Autodesk Fusion 360 part; units mm, degrees
sketch "Sketch1" plane through (0, 0, 0) normal (0, 0, 1) x (1, 0, 0)
  line L0 (0, 0) -> (28, 0)
  line L1 (28, 0) -> (28, 160)
  line L2 (28, 160) -> (0, 160)
  line L3 (0, 160) -> (0, 0) construction
  line L4 (20, 0) -> (20, 160) construction
  line L5 (22.5, 155) -> (25.5, 155)
  line L6 (25.5, 155) -> (25.5, 145)
  line L7 (25.5, 145) -> (22.5, 145)
  line L8 (22.5, 145) -> (22.5, 155)
  line L9 (25.5, 155) -> (25.5, 160) construction
  line L10 (25.5, 155) -> (28, 155) construction
  line L11 (22.5, 135) -> (25.5, 135)
  line L12 (25.5, 135) -> (25.5, 125)
  line L13 (25.5, 125) -> (22.5, 125)
  line L14 (22.5, 125) -> (22.5, 135)
  line L15 (24, 145) -> (24, 135) construction
  line L16 (22.5, 105) -> (22.5, 115)
  line L17 (25.5, 105) -> (22.5, 105)
  line L18 (25.5, 115) -> (25.5, 105)
  line L19 (22.5, 115) -> (25.5, 115)
  line L20 (24, 115) -> (24, 125) construction
  line L21 (25.5, 95) -> (25.5, 85)
  line L22 (25.5, 85) -> (22.5, 85)
  line L23 (22.5, 85) -> (22.5, 95)
  line L24 (22.5, 95) -> (25.5, 95)
  line L25 (24, 95) -> (24, 105) construction
  line L26 (25.5, 95) -> (28, 95) construction
  line L27 (22.5, 75) -> (25.5, 75)
  line L28 (25.5, 75) -> (25.5, 65)
  line L29 (25.5, 65) -> (22.5, 65)
  line L30 (22.5, 65) -> (22.5, 75)
  line L31 (22.5, 55) -> (25.5, 55)
  line L32 (25.5, 55) -> (25.5, 45)
  line L33 (25.5, 45) -> (22.5, 45)
  line L34 (22.5, 45) -> (22.5, 55)
  line L35 (24, 85) -> (24, 75) construction
  line L36 (25.5, 75) -> (28, 75) construction
  line L37 (25.5, 55) -> (28, 55) construction
  line L38 (24, 55) -> (24, 65) construction
  line L39 (25.5, 135) -> (28, 135) construction
  line L40 (25.5, 115) -> (28, 115) construction
  line L41 (22.5, 35) -> (25.5, 35)
  line L42 (25.5, 35) -> (25.5, 25)
  line L43 (25.5, 25) -> (22.5, 25)
  line L44 (22.5, 25) -> (22.5, 35)
  line L45 (25.5, 35) -> (28, 35) construction
  line L46 (24, 45) -> (24, 35) construction
  line L47 (22.5, 15) -> (25.5, 15)
  line L48 (25.5, 15) -> (25.5, 5)
  line L49 (25.5, 5) -> (22.5, 5)
  line L50 (22.5, 5) -> (22.5, 15)
  line L51 (24, 15) -> (24, 25) construction
  line L52 (25.5, 15) -> (28, 15) construction
  line L53 (-25.5, 75) -> (-28, 75) construction
  line L54 (-25.5, 75) -> (-25.5, 65)
  line L55 (-20, 0) -> (-20, 160) construction
  line L56 (-24, 85) -> (-24, 75) construction
  line L57 (-25.5, 115) -> (-28, 115) construction
  line L58 (-22.5, 45) -> (-22.5, 55)
  line L59 (-25.5, 145) -> (-22.5, 145)
  line L60 (-25.5, 135) -> (-28, 135) construction
  line L61 (-22.5, 115) -> (-25.5, 115)
  line L62 (-25.5, 105) -> (-22.5, 105)
  line L63 (-22.5, 65) -> (-22.5, 75)
  line L64 (0, 160) -> (0, 0) construction
  line L65 (-24, 45) -> (-24, 35) construction
  line L66 (-25.5, 135) -> (-25.5, 125)
  line L67 (-28, 160) -> (0, 160)
  line L68 (-25.5, 155) -> (-28, 155) construction
  line L69 (-25.5, 125) -> (-22.5, 125)
  line L70 (-25.5, 55) -> (-28, 55) construction
  line L71 (-24, 15) -> (-24, 25) construction
  line L72 (-22.5, 135) -> (-25.5, 135)
  line L73 (-25.5, 15) -> (-28, 15) construction
  line L74 (-22.5, 75) -> (-25.5, 75)
  line L75 (-25.5, 115) -> (-25.5, 105)
  line L76 (-25.5, 155) -> (-25.5, 145)
  line L77 (-22.5, 105) -> (-22.5, 115)
  line L78 (-24, 115) -> (-24, 125) construction
  line L79 (-25.5, 95) -> (-25.5, 85)
  line L80 (-25.5, 55) -> (-25.5, 45)
  line L81 (-28, 0) -> (-28, 160)
  line L82 (-22.5, 155) -> (-25.5, 155)
  line L83 (-22.5, 85) -> (-22.5, 95)
  line L84 (-24, 95) -> (-24, 105) construction
  line L85 (-25.5, 15) -> (-25.5, 5)
  line L86 (-25.5, 5) -> (-22.5, 5)
  line L87 (-25.5, 155) -> (-25.5, 160) construction
  line L88 (-25.5, 35) -> (-28, 35) construction
  line L89 (-22.5, 25) -> (-22.5, 35)
  line L90 (-22.5, 35) -> (-25.5, 35)
  line L91 (-25.5, 95) -> (-28, 95) construction
  line L92 (-25.5, 25) -> (-22.5, 25)
  line L93 (-22.5, 95) -> (-25.5, 95)
  line L94 (-25.5, 45) -> (-22.5, 45)
  line L95 (-22.5, 125) -> (-22.5, 135)
  line L96 (-22.5, 145) -> (-22.5, 155)
  line L97 (-24, 145) -> (-24, 135) construction
  line L98 (-22.5, 55) -> (-25.5, 55)
  line L99 (-25.5, 65) -> (-22.5, 65)
  line L100 (-25.5, 85) -> (-22.5, 85)
  line L101 (-24, 55) -> (-24, 65) construction
  line L102 (-25.5, 35) -> (-25.5, 25)
  line L103 (0, 0) -> (-28, 0)
  line L104 (-22.5, 15) -> (-25.5, 15)
  line L105 (-22.5, 5) -> (-22.5, 15)
  point P0 (24, 115)
  point P1 (24, 95)
  point P2 (24, 95)
  point P3 (-24, 115)
  point P4 (-24, 95)
  point P5 (-24, 95)
  dimension "d3" = 160
  dimension "d4" = 28
  dimension "d5" = 5
  dimension "d6" = 2.5
  dimension "d7" = 10
  dimension "d8" = 3
  dimension "d9" = 10
extrude "Extrude1" add sketch "Sketch1" along normal blind 3
sketch "Sketch2" plane through (0, 0, 3) normal (0, 0, 1) x (-1, 0, 0)
  line L0 (-22.5, -105) -> (-22.5, -115)
  line L1 (-22.5, -115) -> (-25.5, -115)
  line L2 (-25.5, -115) -> (-25.5, -105)
  line L3 (-25.5, -105) -> (-22.5, -105)
  line L4 (-22.5, -85) -> (-22.5, -95)
  line L5 (-22.5, -95) -> (-25.5, -95)
  line L6 (-25.5, -95) -> (-25.5, -85)
  line L7 (-25.5, -85) -> (-22.5, -85)
  line L8 (-25.5, -145) -> (-22.5, -145)
  line L9 (-22.5, -145) -> (-22.5, -155)
  line L10 (-22.5, -155) -> (-25.5, -155)
  line L11 (-25.5, -155) -> (-25.5, -145)
  line L12 (-25.5, -65) -> (-22.5, -65)
  line L13 (-22.5, -65) -> (-22.5, -75)
  line L14 (-22.5, -75) -> (-25.5, -75)
  line L15 (-25.5, -75) -> (-25.5, -65)
  line L16 (-25.5, -125) -> (-22.5, -125)
  line L17 (-22.5, -125) -> (-22.5, -135)
  line L18 (-22.5, -135) -> (-25.5, -135)
  line L19 (-25.5, -135) -> (-25.5, -125)
  line L20 (-25.5, -25) -> (-22.5, -25)
  line L21 (-22.5, -25) -> (-22.5, -35)
  line L22 (-22.5, -35) -> (-25.5, -35)
  line L23 (-25.5, -35) -> (-25.5, -25)
  line L24 (-25.5, -5) -> (-22.5, -5)
  line L25 (-22.5, -5) -> (-22.5, -15)
  line L26 (-22.5, -15) -> (-25.5, -15)
  line L27 (-25.5, -15) -> (-25.5, -5)
  line L28 (22.5, -115) -> (22.5, -105)
  line L29 (22.5, -105) -> (25.5, -105)
  line L30 (25.5, -105) -> (25.5, -115)
  line L31 (25.5, -115) -> (22.5, -115)
  line L32 (22.5, -15) -> (22.5, -5)
  line L33 (22.5, -5) -> (25.5, -5)
  line L34 (25.5, -5) -> (25.5, -15)
  line L35 (25.5, -15) -> (22.5, -15)
  line L36 (25.5, -25) -> (25.5, -35)
  line L37 (25.5, -35) -> (22.5, -35)
  line L38 (22.5, -35) -> (22.5, -25)
  line L39 (22.5, -25) -> (25.5, -25)
  line L40 (22.5, -85) -> (25.5, -85)
  line L41 (25.5, -85) -> (25.5, -95)
  line L42 (25.5, -95) -> (22.5, -95)
  line L43 (22.5, -95) -> (22.5, -85)
  line L44 (22.5, -65) -> (25.5, -65)
  line L45 (25.5, -65) -> (25.5, -75)
  line L46 (25.5, -75) -> (22.5, -75)
  line L47 (22.5, -75) -> (22.5, -65)
  line L48 (25.5, -55) -> (22.5, -55)
  line L49 (22.5, -55) -> (22.5, -45)
  line L50 (22.5, -45) -> (25.5, -45)
  line L51 (25.5, -45) -> (25.5, -55)
  line L52 (22.5, -155) -> (22.5, -145)
  line L53 (22.5, -145) -> (25.5, -145)
  line L54 (25.5, -145) -> (25.5, -155)
  line L55 (25.5, -155) -> (22.5, -155)
  line L56 (22.5, -135) -> (22.5, -125)
  line L57 (22.5, -125) -> (25.5, -125)
  line L58 (25.5, -125) -> (25.5, -135)
  line L59 (25.5, -135) -> (22.5, -135)
  line L60 (-25.5, -45) -> (-22.5, -45)
  line L61 (-22.5, -45) -> (-22.5, -55)
  line L62 (-22.5, -55) -> (-25.5, -55)
  line L63 (-25.5, -55) -> (-25.5, -45)
  line L64 (-28, 0) -> (-28, -160)
  line L65 (-28, -160) -> (28, -160)
  line L66 (28, -160) -> (28, 0)
  line L67 (28, 0) -> (-28, 0)
Work out the finished part from the listing and answer in its coordinate system (mm). A direction names the side the tool comes from. Give positions to 0.01 mm unless a question says otherwise; leave off trailing zeros. Order: outer loops, then holes, each group sorted by start corner. A loop starts at its lowest first (then second) coordinate and runs counter-clockwise, first axis right, second up.
1. For faces 1 (the flat face through (28, 79, 1)), 2 (the flat face through (25.5, 70, 1)), determine the directions among +Z, -Z, +X, -X, +Y, -Y from which every point of the face is accessible in a straight line to the end or side of a thin tool.
Result sheet:
face 1: +Z, -Z, +X, +Y, -Y
face 2: +Z, -Z
2. Section B-B, the plane z = 2.35 is taken. Give the number of separate pieces and of enclosed holes in the cut face, and give its area (3 significant figures).
Result sheet:
separate pieces: 1
enclosed holes: 16
area: 8,480 mm2
3. A straight line is drawn through the part: L1, parallel to X at y = 88.5, z = 2.7. Find the intervals that lie inside material, in ascending order.
Result sheet:
L1: x = -28 to -25.5, -22.5 to 22.5, 25.5 to 28
4. Section A-A, the plane y = 11 is taken. Determine the outline of the cut face in (x, z), and give its area (3 significant figures).
Result sheet:
outline: (-28, 0) - (-25.5, 0) - (-25.5, 3) - (-28, 3) - close; (-22.5, 0) - (22.5, 0) - (22.5, 3) - (-22.5, 3) - close; (25.5, 0) - (28, 0) - (28, 3) - (25.5, 3) - close
area: 150 mm2
